```python
from build123d import *

# Parameters (mm, degrees)
PAD004_DEPTH    = 8.2
SKETCH014_W     = 28.5
SKETCH014_H     = 6.1
PAD005_DEPTH    = 1.8
SKETCH015_R     = 2.9
POCKET004_DEPTH = 0.6
SKETCH016_W     = 2.05
SKETCH016_H     = 6.1
POCKET005_DEPTH = 1.8
SKETCH018_R     = 1.05
POCKET007_DEPTH = 6


with BuildPart() as part:
    # Sketch013 → Pad004 (new body)
    with BuildSketch(Plane.XY):
        with BuildLine():
            Line((0, 0), (28.5, 0))
            Line((28.5, 0), (28.5, 22.75))
            Line((28.5, 22.75), (14, 22.75))
            Line((14, 22.75), (14, 22.5))
            ThreePointArc((11, 19.5), (13.12132, 20.37868), (14, 22.5))
            Line((11, 19.5), (0, 19.5))
            Line((0, 19.5), (0, 0))
        make_face()
    extrude(amount=PAD004_DEPTH)

    # Sketch014 (on Face9 of Pad004) → Pad005 (join)
    with BuildSketch(Plane.XY.offset(8.2)):
        with Locations((14.25, 9.75)):
            Rectangle(SKETCH014_W, SKETCH014_H)
    extrude(amount=PAD005_DEPTH)

    # Sketch015 (on Face11 of Pad005) → Pocket004 (cut)
    with BuildSketch(Plane.XY.offset(10)):
        with Locations((8.735056, 9.75)):
            Circle(SKETCH015_R)
    extrude(amount=-POCKET004_DEPTH, mode=Mode.SUBTRACT)

    # Sketch016 (on Face10 of Pocket004) → Pocket005 (cut)
    with BuildSketch(Plane.XY.offset(10)):
        with Locations((15.5, 9.75)):
            Rectangle(SKETCH016_W, SKETCH016_H)
        Polygon((21.525, 12.8), (21.525, 6.7), (19.475, 6.7), (19.475, 12.8), (20.5, 12.8), align=None)
        with Locations((25.5, 9.75)):
            Rectangle(SKETCH016_W, SKETCH016_H)
    extrude(amount=-POCKET005_DEPTH, mode=Mode.SUBTRACT)

    # Sketch018 (on Face19 of Clone001) → Pocket007 (cut)
    with BuildSketch(Plane.XY.offset(8.2)):
        with BuildLine():
            Line((14, 22.75), (26.9, 22.75))
            Line((26.9, 22.75), (26.9, 16.25))
            Line((26.355184, 16.25), (26.9, 16.25))
            ThreePointArc((21.044816, 16.25), (23.7, 14.75), (26.355184, 16.25))
            Line((20.45, 16.25), (21.044816, 16.25))
            Line((19.855184, 16.25), (20.45, 16.25))
            ThreePointArc((14.544816, 16.25), (17.2, 14.75), (19.855184, 16.25))
            Line((14, 16.25), (14.544816, 16.25))
            Line((14, 16.25), (14, 22.75))
        make_face()
        with Locations((17.2, 17.85)):
            Circle(SKETCH018_R, mode=Mode.SUBTRACT)
        with Locations((23.7, 17.85)):
            Circle(SKETCH018_R, mode=Mode.SUBTRACT)
    extrude(amount=-POCKET007_DEPTH, mode=Mode.SUBTRACT)


solid = part.part
```
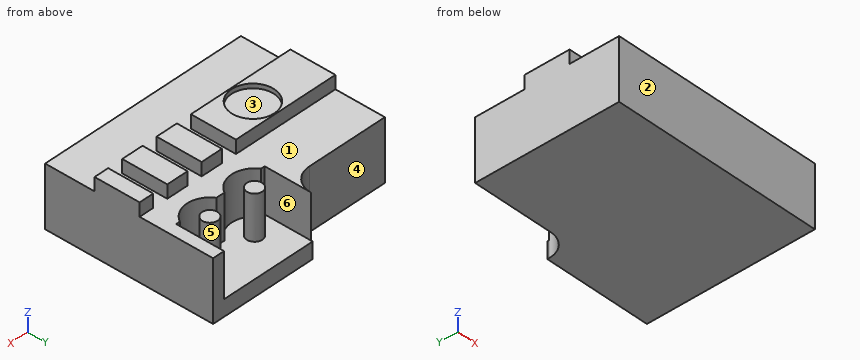
Source: CAD feature listing. Evaluate the final solid. Frame: model axes, mm. Face numbers are marked on the shaded views. A direction names the side the tool comes from. Coordinates: 2 decimals unless noted, no trailing zeros. Order: outer loops, then holes, each group sorted by start corner. A loop starts at its lowest first (then second) coordinate and runs counter-clockwise, first axis right, second up. Notation, with made-up numbers: M -5,18.25 L 10,18.25 A17 ccw 10,50.25 Z; hole C 82,17.5 d8. An arc over 180 degrees is marked long. Write each question's results on one line, items separated by ' | '. Start each with the question number.
1) Contact query for flat-ended pins moving along their axis: pin 1 Ø1 at (x, y) = (19.5, 12.5) entering from +Z; pin 2 Ø2 at (x, z) = (22.5, 9.5) entering from -Y; pin 3 Ø1.7 at (x, y) = (9, 10) entering from +Z; pin 4 Ø4 at (x, z) = (4, 5) entering from +Y. Output: stop coordinate, or through.
2) Section query D-D (z = 0.75). Return the cut outline in (x, y), plus the area to 3 significant figures.
3) Access query for the marked faces 4, 5 and 6. Directions: +Z, -Z, +X, -X, +Y, -Y. A direction counts if a zero-diameter tool reaches every point of the face in a straight line with its end or side. Return the directions, or none.
4) Section query B-B (y = 17.85). Return the cut outline in (x, z).
5) Section query C-C (x = 23.7). Return the cut outline in (y, z), plus the area to 3 significant figures.
6) Line query: line 1 (Y direction, x = 23.75, z = 4); line 2 (Y direction, x = 6.5, z = 7.5); line 3 (Z direction, x = 21.5, y = 19). Output: solid intervals per line, ascending. Write a range as from..to.
7) Section query A-A (z = 3.5). Return the cut outline in (x, y), plus the area to 3 significant figures.
8) Draft query along Y for the marked faces 1, 2 and 3. Return one class per face: released by +Y, released by -Y, zero draft, split by the parting line, or undercut.
Answers:
1) pin 1: stops at z = 10 | pin 2: stops at y = 6.7 | pin 3: stops at z = 9.4 | pin 4: stops at y = 19.5
2) outline: M 0,0 L 28.5,0 L 28.5,22.75 L 14,22.75 L 14,22.5 A3 cw 11,19.5 L 0,19.5 Z | area: 605 mm^2
3) face 4: +Z, -Z, -X, +Y | face 5: +Z | face 6: +Z, +Y
4) outline: M 0,0 L 28.5,0 L 28.5,8.2 L 26.9,8.2 L 26.9,2.2 L 24.75,2.2 L 24.75,8.2 L 22.65,8.2 L 22.65,2.2 L 18.25,2.2 L 18.25,8.2 L 16.15,8.2 L 16.15,2.2 L 14,2.2 L 14,8.2 L 0,8.2 Z
5) outline: M 0,0 L 22.75,0 L 22.75,2.2 L 18.9,2.2 L 18.9,8.2 L 16.8,8.2 L 16.8,2.2 L 14.75,2.2 L 14.75,8.2 L 12.8,8.2 L 12.8,10 L 6.7,10 L 6.7,8.2 L 0,8.2 Z | area: 162 mm^2
6) line 1: y = 0..14.75, 16.8..18.9 | line 2: y = 0..19.5 | line 3: z = 0..2.2
7) outline: M 0,0 L 28.5,0 L 28.5,22.75 L 26.9,22.75 L 26.9,16.25 L 26.36,16.25 A3.1 cw 21.04,16.25 L 19.86,16.25 A3.1 cw 14.54,16.25 L 14,16.25 L 14,22.5 A3 cw 11,19.5 L 0,19.5 Z; C 17.2,17.85 d2.1; C 23.7,17.85 d2.1 | area: 517 mm^2
8) face 1: zero draft | face 2: released by -Y | face 3: undercut
